Read the model definition and answer for the solid it produces. Units are mm, in the model's axes. Face numbers are marked on the shaded views. A direction names the side the tool comes from. Give positions to 0.01 mm unless a question says otherwise; leave off trailing zeros. Loops run counter-clockwise (first coordinate to the right, second up) from the corner with the lowest first, then second, coordinate; pieces in that order, holes last. Notation, with made-up numbers: M 66,27 L 95,27 A17 ccw 95,45 Z; hole C 40.25,40 d5. An arc over 180 degrees is marked long. Return JSON: item names as keys, results as strings. Group by question number.
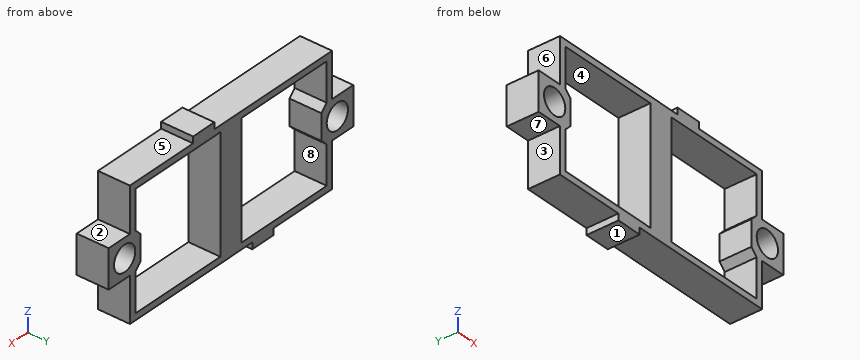
```python
from build123d import *

# Parameters (mm, degrees)
SKETCH1_R           = 12.7
BOSS_EXTRUDE2_DEPTH = 31.75


with BuildPart() as part:
    # Sketch1 → Boss-Extrude2 (new body)
    with BuildSketch(Plane(origin=(0, 0, 0), x_dir=(1, 0, 0), z_dir=(0, 1, 0))):
        Polygon((95.25, 127), (241.3, 127), (241.3, 82.55), (266.7, 82.55), (266.7, 44.45), (241.3, 44.45), (241.3, 0), (165.851748879, 0), (165.851748879, -6.35), (140.451748879, -6.35), (140.451748879, 0), (0, 0), (0, 44.45), (-25.4, 44.45), (-25.4, 82.55), (0, 82.55), (0, 127), (69.85, 127), (69.85, 133.35), (95.25, 133.35), align=None)
        with Locations(Location((247.65, 63.5, 0), (0, 0, 270))):
            Circle(SKETCH1_R, mode=Mode.SUBTRACT)
        with Locations(Location((-6.35, 63.5, 0), (0, 0, 270))):
            Circle(SKETCH1_R, mode=Mode.SUBTRACT)
        Polygon((6.35, 82.55), (12.7, 76.2), (12.7, 50.8), (6.35, 44.45), (6.35, 6.35), (107.95, 6.35), (107.95, 120.65), (6.35, 120.65), align=None, mode=Mode.SUBTRACT)
        Polygon((234.95, 82.55), (228.6, 76.2), (228.6, 50.8), (234.95, 44.45), (234.95, 6.35), (133.35, 6.35), (133.35, 120.65), (234.95, 120.65), align=None, mode=Mode.SUBTRACT)
    extrude(amount=BOSS_EXTRUDE2_DEPTH)


solid = part.part
```
1. Find section B-B (z = -99). Write down the section's boundary in (x, y).
2. Find section C-C (y = 20). State how many separate pieces and enclosed holes the cut face has, and give its area (3 significant figures).
3. Straight lines are drawn through the part: line 1 along X through (y, z) = (13, -63.5); line 2 along X through (y, z) = (2.5, -119.5); line 3 along Z through (x, y) = (47.5, 30.5). For each, find the intervals that lie inside material, in ascending order.
4. The mould has two halves that part along Z. Classify the marked faces 1, 2, 3 and 4: +Z half, -Z half, draft (parallel to the pull), parting line (faces both ways), or undercut.
5. Find section D-D (x = 27). Write down the section's boundary in (y, z), and give its area (3 significant figures).
6. Find section A-A (x = 89). Write down the section's boundary in (y, z), and give its area (3 significant figures).
7. Flat-ended cylindrical pins translate along their axes: P1, Ø1.5, axis at y = 3.5, z = -93.5, coming from the -X side; P2, Ø6, axis at x = 111.5, y = 15.5, coming from the -Z side; P3, Ø4, axis at x = 137, z = -81, coming from the +Y side; P4, Ø1.5, axis at x = 119.5, y = 22, coming from the +Z side. Find the tip coordinate at first contact, or state that the pin passes through.
8. For the marked faces 5, 6, 7 and 8, determine the directions among +Z, -Z, +X, -X, +Y, -Y from which every point of the face is accessible in a straight line to the end or side of a thin tool.
Result:
{
 "1": {"outline": "M 0,0 L 6.35,0 L 6.35,31.75 L 0,31.75 Z; M 107.95,0 L 133.35,0 L 133.35,31.75 L 107.95,31.75 Z; M 234.95,0 L 241.3,0 L 241.3,31.75 L 234.95,31.75 Z"},
 "2": {"separate pieces": "1", "enclosed holes": "4", "area": "9,070 mm2"},
 "3": {"line 1": "x = -25.4 to -19.05, 6.35 to 12.7, 107.95 to 133.35, 228.6 to 234.95, 260.35 to 266.7", "line 2": "x = 0 to 6.35, 107.95 to 133.35, 234.95 to 241.3", "line 3": "z = -127 to -120.65, -6.35 to 0"},
 "4": {"face 1": "-Z half", "face 2": "+Z half", "face 3": "draft", "face 4": "undercut"},
 "5": {"outline": "M 0,-127 L 31.75,-127 L 31.75,-120.65 L 0,-120.65 Z; M 0,-6.35 L 31.75,-6.35 L 31.75,0 L 0,0 Z", "area": "403 mm2"},
 "6": {"outline": "M 0,-133.35 L 31.75,-133.35 L 31.75,-120.65 L 0,-120.65 Z; M 0,-6.35 L 31.75,-6.35 L 31.75,0 L 0,0 Z", "area": "605 mm2"},
 "7": {"P1": "stops at x = 0", "P2": "stops at z = -127", "P3": "passes through", "P4": "stops at z = 0"},
 "8": {"face 5": "+Z, +X, +Y, -Y", "face 6": "+Z, -X, +Y, -Y", "face 7": "-Z, -X, +Y, -Y", "face 8": "+Y, -Y"}
}
